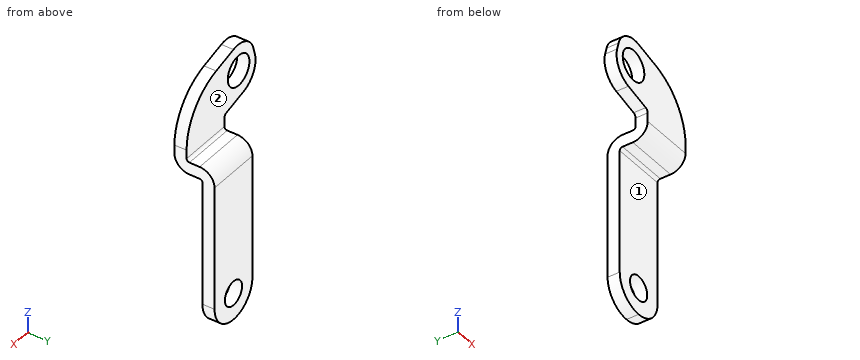
```python
from build123d import *

# Parameters (mm, degrees)
SKETCH1_R                    = 4
BASE_FLANGE1_DEPTH           = 3.175
EDGE_FLANGE1_STRIP_W         = 14.1732
EDGE_FLANGE1_STRIP_H         = 3.175
EDGE_FLANGE1_STRIP_CUT_DEPTH = 14
EDGE_FLANGE1_DEPTH           = 14
EDGE_FLANGE2_STRIP_W         = 14.1732
EDGE_FLANGE2_STRIP_H         = 3.175
EDGE_FLANGE2_STRIP_CUT_DEPTH = 14
EDGE_FLANGE2_DEPTH           = 14
SKETCH17_R                   = 3.175
CUT_EXTRUDE1_DEPTH           = 3.175


# Sheet-metal steps are written as plain solids
with BuildPart() as part:
    # Sketch1 → Base-Flange1 (new body)
    with BuildSketch(Plane(origin=(0, 0, 0), x_dir=(1, 0, 0), z_dir=(0, 1, 0))):
        with BuildLine():
            Line((19.250001318, 12.5), (5.250001318, 12.5))
            Line((5.250001318, 12.5), (5.250001318, 9.5))
            ThreePointArc((5.250001318, 9.5), (5.046855339, 8.895828112), (4.519953978, 8.537126404))
            Line((4.519953978, 8.537126404), (-1.889668619, 6.740115171))
            ThreePointArc((-1.889668619, 6.740115171), (-5.500391492, 3.902688152), (-6.047194235, -0.656842363))
            Line((-6.047194235, -0.656842363), (-5.507288915, -2.582589555))
            ThreePointArc((-5.507288915, -2.582589555), (-2.669861896, -6.193312428), (1.889668619, -6.740115171))
            Line((1.889668619, -6.740115171), (8.299291215, -4.943103937))
            ThreePointArc((8.299291215, -4.943103937), (16.202811625, 0.437421682), (19.250001318, 9.5))
            Line((19.250001318, 9.5), (19.250001318, 12.5))
        make_face()
        with Locations(Location((0, 0, 0), (0, 0, 270))):
            Circle(SKETCH1_R, mode=Mode.SUBTRACT)
    extrude(amount=-BASE_FLANGE1_DEPTH)

    # Edge-Flange1 strip (across the edge) → Edge-Flange1 strip cut (cut)
    with BuildSketch(Plane(origin=(19.250001318, 0, -12.5), x_dir=(0, 0, 1), z_dir=(-1, 0, 0))):
        with Locations((-6.35, -1.5875)):
            Rectangle(EDGE_FLANGE1_STRIP_W, EDGE_FLANGE1_STRIP_H)
    extrude(amount=EDGE_FLANGE1_STRIP_CUT_DEPTH, mode=Mode.SUBTRACT)

    # Edge-Flange1 section (across the edge) → Edge-Flange1 (add)
    with BuildSketch(Plane(origin=(19.250001318, 0, -12.5), x_dir=(0, 0, 1), z_dir=(-1, 0, 0))):
        with BuildLine():
            Line((-3.175, 0.7366), (-3.175, 7.324994814))
            Line((-3.175, 7.324994814), (0, 7.324994814))
            Line((0, 7.324994814), (0, 0.7366))
            ThreePointArc((0, 0.7366), (0.215745145, 0.215745145), (0.7366, 0))
            Line((0.7366, 0), (0.7366, -3.175))
            ThreePointArc((0.7366, -3.175), (-2.029318885, -2.029318885), (-3.175, 0.7366))
        make_face()
    extrude(amount=EDGE_FLANGE1_DEPTH)

    # Edge-Flange2 strip (across the edge) → Edge-Flange2 strip cut (cut)
    with BuildSketch(Plane(origin=(5.250001318, 7.324994814, -15.675), x_dir=(0, -1, 0), z_dir=(1, 0, 0))):
        with Locations((-3.175, -1.5875)):
            Rectangle(EDGE_FLANGE2_STRIP_W, EDGE_FLANGE2_STRIP_H)
    extrude(amount=EDGE_FLANGE2_STRIP_CUT_DEPTH, mode=Mode.SUBTRACT)

    # Edge-Flange2 section (across the edge) → Edge-Flange2 (add)
    with BuildSketch(Plane(origin=(5.250001318, 7.324994814, -15.675), x_dir=(0, -1, 0), z_dir=(1, 0, 0))):
        with BuildLine():
            Line((0, 0.7366), (0, 40.174998631))
            Line((0, 40.174998631), (3.175, 40.174998631))
            Line((3.175, 40.174998631), (3.175, 0.7366))
            ThreePointArc((3.175, 0.7366), (3.390745145, 0.215745145), (3.9116, 0))
            Line((3.9116, 0), (3.9116, -3.175))
            ThreePointArc((3.9116, -3.175), (1.145681115, -2.029318885), (0, 0.7366))
        make_face()
    extrude(amount=EDGE_FLANGE2_DEPTH)

    # Sketch17 → Cut-Extrude1 (cut)
    with BuildSketch(Plane(origin=(0, 7.324994814, 0), x_dir=(1, 0, 0), z_dir=(0, 1, 0))):
        with BuildLine():
            ThreePointArc((5.250001318, 48.849998631), (7.30025385, 53.7997461), (12.250001318, 55.849998631))
            Line((12.250001318, 55.849998631), (5.250001318, 55.849998631))
            Line((5.250001318, 55.849998631), (5.250001318, 48.849998631))
        make_face()
        with BuildLine():
            ThreePointArc((12.250001318, 55.849998631), (17.199748787, 53.7997461), (19.250001318, 48.849998631))
            Line((19.250001318, 48.849998631), (19.250001318, 55.849998631))
            Line((19.250001318, 55.849998631), (12.250001318, 55.849998631))
        make_face()
        with Locations(Location((12.250001318, 48.849998631, 0), (0, 0, 270))):
            Circle(SKETCH17_R)
    extrude(amount=-CUT_EXTRUDE1_DEPTH, mode=Mode.SUBTRACT)


solid = part.part
```
Source: CAD feature listing. Evaluate the final solid. Frame: model axes, mm. Face numbers are marked on the shaded views. Give positions to 0.01 mm unless a question says otherwise; leave off trailing zeros. Order: outer loops, then holes, each group sorted by start corner. A loop starts at its lowest first (then second) coordinate and runs counter-clockwise, first axis right, second up.
(1) Section query D-D (z = -24.5). Return the cut outline in (x, y) (3 decimals).
(2) Section query C-C (y = -0.75). Return the cut outline in (x, z).
(3) Contact query for flat-ended pins moving along their axis: P1, Ø4, axis at x = 6, y = 1.5, coming from the -Z side; P2, Ø10, axis at x = 12.25, z = -48.85, coming from the -Y side; P3, Ø6.5, axis at x = 0, z = 0, coming from the -Y side; P4, Ø3, axis at x = 9, y = 2.5, coming from the +Z side. Output: stop coordinate, or through.
(4) Section query B-B (x = 0). Return the cut outline in (y, z) (3 decimals).
(5) Pull-direction query (Y, two-part tool) for the marked faces 1 and 2; classes: +Y half, -Y half, draft (parallel to the pull), parting line (faces both ways), or undercut.
(6) Section query A-A (z = 0). Return the cut outline in (x, y) (3 decimals).
(7) Material intervals for line 1 along Z through (x, y) = (14, 4.5); line 2 along X through (y, z) = (5.5, -20); line 3 along Y through (x, z) = (13, -20) (3 decimals), sorted ascending.
Outcome:
1. outline: (5.25, 4.15) - (19.25, 4.15) - (19.25, 7.325) - (5.25, 7.325) - close
2. outline: (-6.05, 0.66) arc R6 ccw to (-1.89, -6.74) - (4.52, -8.54) arc R1 cw to (5.25, -9.5) - (5.25, -15.38) - (19.25, -15.38) - (19.25, -9.5) arc R15 ccw to (8.3, 4.94) - (1.89, 6.74) arc R6 ccw to (-5.51, 2.58) - close; hole circle Ø8 at (0, 0)
3. P1: stops at z = -15.68
3. P2: stops at y = 4.15
3. P3: passes through
3. P4: stops at z = -12.5
4. outline: (-3.175, -7.27) - (0, -7.27) - (0, -4) - (-3.175, -4) - close; (-3.175, 4) - (0, 4) - (0, 6.957) - (-3.175, 6.957) - close
5. face 1: -Y half
5. face 2: +Y half
6. outline: (-6.192, -3.175) - (-4, -3.175) - (-4, 0) - (-6.192, 0) - close; (4, -3.175) - (15.858, -3.175) - (15.858, 0) - (4, 0) - close
7. line 1: z = -55.63 to -51.5, -46.2 to -12.65
7. line 2: x = 5.25 to 19.25
7. line 3: y = 4.15 to 7.325
